Model file for the job. Use its own axes, mm. Coordinates: 2 decimals unless noted, no trailing zeros. Loops run counter-clockwise (first coordinate to the right, second up) from the corner with the lowest first, then second, coordinate; pieces in that order, holes last.
from build123d import *

# Parameters (mm, degrees)
EXTRUDE_1_DEPTH     = 5
FILLET_1_R          = 40
FILLET_2_R          = 5
SKETCH_2_R          = 2
CUT_EXTRUDE_1_DEPTH = 5
FILLET_3_R          = 35
SKETCH_3_R          = 9
CUT_EXTRUDE_2_DEPTH = 99.12125789
SKETCH_4_R          = 2
CUT_EXTRUDE_3_DEPTH = 99.12125789


with BuildPart() as part:
    # 草图1 → 凸台-拉伸1 (new body)
    with BuildSketch(Plane(origin=(0, 0, 0), x_dir=(1, 0, 0), z_dir=(0, 1, 0))):
        Polygon((-89.625, 35.375), (10.375, 35.375), (10.375, -39.625), (-19.625, -39.625), (-19.625, 15.375), (-89.625, 15.375), align=None)
    extrude(amount=EXTRUDE_1_DEPTH)

    # 圆角1
    fillet_1_edges = [part.edges().sort_by_distance(p)[0] for p in [
        (-19.625, 2.5, -15.375),
    ]]
    fillet(fillet_1_edges, radius=FILLET_1_R)

    # 圆角2
    fillet_2_edges = [part.edges().sort_by_distance(p)[0] for p in [
        (-89.625, 2.5, -35.375),
        (10.375, 2.5, 39.625),
        (-19.625, 2.5, 39.625),
        (-89.625, 2.5, -15.375),
    ]]
    fillet(fillet_2_edges, radius=FILLET_2_R)

    # 草图2 → 切除-拉伸1 (cut)
    with BuildSketch(Plane(origin=(0, 5, 0), x_dir=(1, 0, 0), z_dir=(0, 1, 0))):
        with Locations(Location((-14.625, -29.625, 0), (0, 0, 270))):
            Circle(SKETCH_2_R)
        with Locations(Location((5.375, -29.625, 0), (0, 0, 270))):
            Circle(SKETCH_2_R)
        with Locations(Location((5.375, -19.625, 0), (0, 0, 270))):
            Circle(SKETCH_2_R)
        with Locations(Location((-14.625, -19.625, 0), (0, 0, 270))):
            Circle(SKETCH_2_R)
    extrude(amount=-CUT_EXTRUDE_1_DEPTH, mode=Mode.SUBTRACT)

    # 圆角3
    fillet_3_edges = [part.edges().sort_by_distance(p)[0] for p in [
        (10.375, 2.5, -35.375),
    ]]
    fillet(fillet_3_edges, radius=FILLET_3_R)

    # 草图3 → 切除-拉伸2 (cut, through all)
    with BuildSketch(Plane(origin=(0, 5, 0), x_dir=(1, 0, 0), z_dir=(0, 1, 0))):
        with Locations(Location((-19.625, 20.375, 0), (0, 0, 270))):
            Circle(SKETCH_3_R)
        with Locations(Location((-4.625, -4.625, 0), (0, 0, 270))):
            Circle(SKETCH_3_R)
    extrude(amount=-CUT_EXTRUDE_2_DEPTH, mode=Mode.SUBTRACT)

    # 草图4 → 切除-拉伸3 (cut, through all)
    with BuildSketch(Plane(origin=(0, 5, 0), x_dir=(1, 0, 0), z_dir=(0, 1, 0))):
        with Locations(Location((-79.625, 25.375, 0), (0, 0, 270))):
            Circle(SKETCH_4_R)
        with Locations(Location((-54.625, 25.375, 0), (0, 0, 270))):
            Circle(SKETCH_4_R)
    extrude(amount=-CUT_EXTRUDE_3_DEPTH, mode=Mode.SUBTRACT)


solid = part.part
Q1. Slice it at D-D (z = 2). List the corners of the cut face in (x, y) (1 decimal).
Answers:
outline: (-26.6, 0) - (-13.2, 0) - (-13.2, 5) - (-26.6, 5) - close; (4, 0) - (10.4, 0) - (10.4, 5) - (4, 5) - close
Q2. Slice it at A-A (z = -25). List the corners of the cut face in (x, y) (3 decimals).
Answers:
outline: (-89.625, 0) - (-81.59, 0) - (-81.59, 5) - (-89.625, 5) - close; (-77.66, 0) - (-56.59, 0) - (-56.59, 5) - (-77.66, 5) - close; (-52.66, 0) - (-27.346, 0) - (-27.346, 5) - (-52.66, 5) - close; (-11.904, 0) - (0.247, 0) - (0.247, 5) - (-11.904, 5) - close
Q3. Slice it at C-C (y = 4.2). Count the separate pieces of the cut face and the enclosed holes in it, and give its area (3 significant figures).
Answers:
separate pieces: 1
enclosed holes: 8
area: 3,120 mm2
Q4. Drill centre lines: line 1 (Z direction, x = -4, y = 1.25) (3 decimals); line 2 (Z direction, x = -67, y = 2.6) (3 decimals); line 3 (X direction, y = 3.55, z = 33.5) (3 decimals). Where is each one in solid material? Low to high.
Answers:
line 1: z = -28.652 to -4.353, 13.603 to 39.625
line 2: z = -35.375 to -15.375
line 3: x = -19.625 to 10.375
Q5. Slice it at B-B (x = -6). List the corners of the cut face in (y, z) (3 decimals), and give its area (3 significant figures).
Answers:
outline: (0, -30.008) - (5, -30.008) - (5, -4.269) - (0, -4.269) - close; (0, 13.519) - (5, 13.519) - (5, 39.625) - (0, 39.625) - close
area: 259 mm2
Q6. Mould opens along Z. For faces 1 (the flat face through (-55, 2, -35.375)), 2 (the flat face through (-19.625, 2, 30)), 3 (the cylindrical face through (6.727, 2.535, 18.151)) say: +Z half, -Z half, draft (parallel to the pull), parting line (faces both ways), or undercut.
Answers:
face 1: -Z half
face 2: draft
face 3: undercut
Q7. Flat gauge pins, fed straight in: P1, Ø1.5, axis at y = 4, z = 6.5, coming from the -X side; P2, Ø3, axis at x = -6.5, y = 4, coming from the -Z side; P3, Ø5, axis at x = 5.375, z = 19.625, coming from the -Y side; P4, Ø1.5, axis at y = 3, z = -5.5, coming from the -X side. Where does each tip first touch, or does it go through?
Answers:
P1: stops at x = -24.36
P2: stops at z = -31.17
P3: stops at y = 0
P4: stops at x = -34.19
